Verification items for the finished model (mm, model axes). Face numbers are marked on the shaded views. A direction names the side the tool comes from. Give positions to 0.01 mm unless a question says otherwise; leave off trailing zeros. Loops run counter-clockwise (first coordinate to the right, second up) from the corner with the lowest first, then second, coordinate; pieces in that order, holes last. Notation, with made-up numbers: (23, 83.5) -> (48, 83.5) arc R17 cw to (48, 94.5) -> close; hole circle Ø5 at (83, 37.25). An arc over 180 degrees is marked (long way). Answer in a Markdown table with one row per item. Add a question column.
Q1. Set-up check for the marked faces 1, 2 and 3: record each of +Z, -Z, +X, -X, +Y, -Y from which the full face is reachable in a straight line by a thin tool's end or side.
Q2. Material ranges on probe 1 along Y at (x, z) = (0, 0.25); probe 2 along Y at (x, z) = (0, 0.15); probe 3 along Z at (x, y) = (-2, 2), recorded low to high.
Q3. Section check D-D on z = 21.5. Enter the section's corners in (x, y).
Q4. Section check C-C on z = 4. Enter the section's corners in (x, y).
Q5. Section check A-A on y = 0. Enter the section's corners in (x, z).
Q6. Gauge pin test, flat ends, axial feed: P1, Ø3, axis at x = 0, z = 11, coming from the -Y side; P2, Ø4, axis at y = 0.5, z = 7, coming from the -X side; P3, Ø1.2, axis at x = 0, z = 14.5, coming from the +Y side; P4, Ø3, axis at x = 6.5, z = 23.5, coming from the -Y side. Record the tip position at first contact, or that the pin passes through.
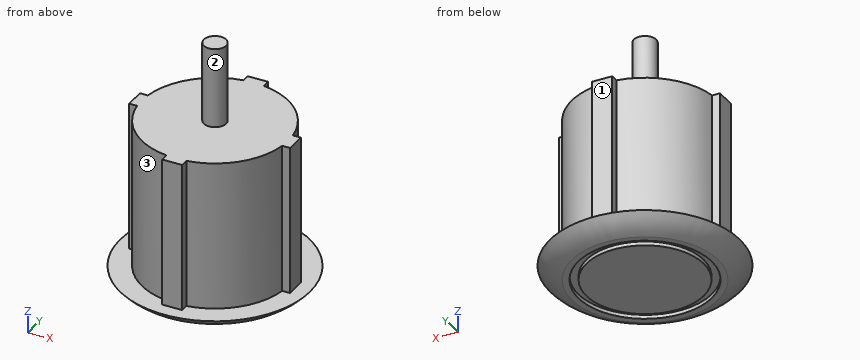
```python
from build123d import *

# Parameters (mm, degrees)
SKETCH_1_R               = 9.1
EXTRUDE_1_DEPTH          = 20.4
SKETCH_3_R               = 8.294737136
SKETCH_3_R_2             = 7.294737136
CUT_EXTRUDE_1_DEPTH      = 0.5
SKETCH_4_W               = 2.5
SKETCH_4_H               = 2
EXTRUDE_2_DEPTH          = 18.6
PATTERN_CIRCULAR_1_COUNT = 4
SKETCH_5_R               = 1.4
EXTRUDE_3_DEPTH          = 10


with BuildPart() as part:
    # 草图1 → 凸台-拉伸1 (new body)
    with BuildSketch(Plane.XY):
        Circle(SKETCH_1_R)
    extrude(amount=EXTRUDE_1_DEPTH)

    # 草图2 → 旋转1 (revolve)
    with BuildSketch(Plane(origin=(0, 0, 0), x_dir=(0, 0, -1), z_dir=(1, 0, 0)), mode=Mode.PRIVATE) as revolve_1_sk:
        with BuildLine():
            Line((-1.8, 9.1), (-1.8, 11.8))
            ThreePointArc((-1.8, 11.8), (-0.714004188, 10.573997208), (0, 9.1))
            Line((0, 9.1), (-1.8, 9.1))
        make_face()
    revolve(revolve_1_sk.sketch.rotate(Axis((0, 0, 20.4), (0, 0, -1)), 270), axis=Axis((0, 0, 20.4), (0, 0, -1)))

    # 草图3 → 切除-拉伸1 (cut)
    with BuildSketch(Plane(origin=(0, 0, 0), x_dir=(-1, 0, 0), z_dir=(0, 0, -1))):
        Circle(SKETCH_3_R)
        Circle(SKETCH_3_R_2, mode=Mode.SUBTRACT)
    extrude(amount=-CUT_EXTRUDE_1_DEPTH, mode=Mode.SUBTRACT)

    # 草图4 → 凸台-拉伸2 (add)
    with BuildSketch(Plane.XY.offset(20.4)):
        with Locations((0, 9)):
            Rectangle(SKETCH_4_W, SKETCH_4_H)
    extrude_2 = extrude(amount=-EXTRUDE_2_DEPTH)

    # 阵列(圆周)1: 凸台-拉伸2 ×4 about axis
    pattern_circular_1_axis = Axis((0, 0, 0), (0, 0, 1))
    for i in range(1, PATTERN_CIRCULAR_1_COUNT):
        add(extrude_2.rotate(pattern_circular_1_axis, i * 360 / PATTERN_CIRCULAR_1_COUNT))

    # 草图5 → 凸台-拉伸3 (add)
    with BuildSketch(Plane.XY.offset(20.4)):
        Circle(SKETCH_5_R)
    extrude(amount=EXTRUDE_3_DEPTH)


solid = part.part
```
Taken from the geometry:
| question | item | result |
|---|---|---|
| 1 | face 1 | +Z, +X, -X, +Y |
| 1 | face 2 | +Z |
| 1 | face 3 | +Z, -X, -Y |
| 2 | probe 1 | y = -9.74 to -8.29, -7.29 to 7.29, 8.29 to 9.74 |
| 2 | probe 2 | y = -9.51 to -8.29, -7.29 to 7.29, 8.29 to 9.51 |
| 2 | probe 3 | z = 0 to 20.4 |
| 3 | outline | circle Ø2.8 at (0, 0) |
| 4 | outline | (-10, -1.25) -> (-9.01, -1.25) arc R9.1 ccw to (-1.25, -9.01) -> (-1.25, -10) -> (1.25, -10) -> (1.25, -9.01) arc R9.1 ccw to (9.01, -1.25) -> (10, -1.25) -> (10, 1.25) -> (9.01, 1.25) arc R9.1 ccw to (1.25, 9.01) -> (1.25, 10) -> (-1.25, 10) -> (-1.25, 9.01) arc R9.1 ccw to (-9.01, 1.25) -> (-10, 1.25) -> close |
| 5 | outline | (-11.8, 1.8) arc R6 ccw to (-9.1, 0) -> (-8.29, 0) -> (-8.29, 0.5) -> (-7.29, 0.5) -> (-7.29, 0) -> (7.29, 0) -> (7.29, 0.5) -> (8.29, 0.5) -> (8.29, 0) -> (9.1, 0) arc R6 ccw to (11.8, 1.8) -> (10, 1.8) -> (10, 20.4) -> (1.4, 20.4) -> (1.4, 30.4) -> (-1.4, 30.4) -> (-1.4, 20.4) -> (-10, 20.4) -> (-10, 1.8) -> close |
| 6 | P1 | stops at y = -10 |
| 6 | P2 | stops at x = -10 |
| 6 | P3 | stops at y = 10 |
| 6 | P4 | passes through |
